from build123d import *

# Parameters (mm, degrees)
F1_DEPTH = 22
F3_DEPTH = 2
F5_DEPTH = 25
F7_DEPTH = 25


with BuildPart() as f1:
    # F0 (on Front) → F1 (new body, symmetric)
    with BuildSketch(Plane.XZ):
        with BuildLine():
            Line((-40, 0), (-0.4058661959, 0))
            ThreePointArc((-0.4058661959, 0), (-0.0297944203, 0.073409465), (0.2910628996, 0.2828599608))
            Line((0.2910628996, 0.2828599608), (1.7669371004, 1.7171400392))
            ThreePointArc((1.7669371004, 1.7171400392), (2.0877944203, 1.926590535), (2.4638661959, 2))
            Line((2.4638661959, 2), (26.037, 2))
            ThreePointArc((26.037, 2), (27.9687843496, 2.7891547709), (28.7954749436, 4.705176349))
            Line((28.7954749436, 4.705176349), (29.016465998, 16.0310205539))
            ThreePointArc((29.016465998, 16.0310205539), (28.8276722638, 16.8546583092), (28.2736767263, 17.4927109486))
            Line((28.2736767263, 17.4927109486), (27.3333525812, 18.1512658075))
            Line((27.3333525812, 18.1512658075), (26.1860444646, 16.5130704329))
            Line((26.1860444646, 16.5130704329), (26.8254471929, 16.0652655182))
            Line((26.8254471929, 16.0652655182), (26.037, 4))
            Line((26.037, 4), (1.4428661959, 4))
            ThreePointArc((1.4428661959, 4), (1.0667944203, 3.926590535), (0.7459371004, 3.7171400392))
            Line((0.7459371004, 3.7171400392), (-0.7299371004, 2.2828599608))
            ThreePointArc((-0.7299371004, 2.2828599608), (-1.0507944203, 2.073409465), (-1.4268661959, 2))
            Line((-1.4268661959, 2), (-40, 2))
            Line((-40, 2), (-40, 0))
        make_face()
    extrude(amount=F1_DEPTH, both=True)

    # F2 (on face) → F3 (join)
    with BuildSketch(Plane.XY.offset(2)):
        with BuildLine():
            Line((-50, 12), (-50, -12))
            ThreePointArc((-50, -12), (-47.0710678119, -19.0710678119), (-40, -22))
            Line((-40, -22), (-40, 22))
            ThreePointArc((-40, 22), (-47.0710678119, 19.0710678119), (-50, 12))
        make_face()
    extrude(amount=-F3_DEPTH)

    # F4 (on face) → F5 (cut)
    with BuildSketch(Plane.XY.offset(2)):
        with BuildLine():
            ThreePointArc((-40.35, -11.789), (-42.6, -14.039), (-40.35, -16.289))
            Line((-40.35, -16.289), (-20.35, -16.289))
            ThreePointArc((-20.35, -16.289), (-18.1, -14.039), (-20.35, -11.789))
            Line((-20.35, -11.789), (-40.35, -11.789))
        make_face()
        with BuildLine():
            ThreePointArc((-40.35, 16.289), (-42.6, 14.039), (-40.35, 11.789))
            Line((-40.35, 11.789), (-20.35, 11.789))
            ThreePointArc((-20.35, 11.789), (-18.1, 14.039), (-20.35, 16.289))
            Line((-20.35, 16.289), (-40.35, 16.289))
        make_face()
    extrude(amount=-F5_DEPTH, mode=Mode.SUBTRACT)

    # F6 (on face) → F7 (cut)
    with BuildSketch(Plane(origin=(28.6927430868, 0, -0.5598557981), x_dir=(0, 1, 0), z_dir=(0.9998096932, 0, -0.0195083911))):
        with BuildLine():
            Line((-9.9999997095, 13.096034309), (-17.9999997095, 13.096034309))
            ThreePointArc((-17.9999997095, 13.096034309), (-20, 11.0960344543), (-18, 9.096034309))
            Line((-18, 9.096034309), (-9.9999997095, 9.096034309))
            ThreePointArc((-9.9999997095, 9.096034309), (-7.9999997095, 11.096034309), (-9.9999997095, 13.096034309))
        make_face()
    extrude(amount=-F7_DEPTH, mode=Mode.SUBTRACT)


solid = f1.part
Check sheet for the modelled part. Datum: model origin and axes. Units: mm. A direction names the side the tool comes from. Give positions to 0.01 mm unless a question says otherwise; leave off trailing zeros. Loops run counter-clockwise (first coordinate to the right, second up) from the corner with the lowest first, then second, coordinate; pieces in that order, holes last. Notation, with made-up numbers: M -36,48.25 L -21,48.25 A24 ccw -21,67.25 Z; hole C -31.75,-11 d2. An arc over 180 degrees is marked long. Answer as a JSON object with one key per item and string values. Group by question number.
Q1. Cross-section at B-B on x = -41.5. Record the cut outline in (y, z).
Q2. Cross-section at A-A on y = 10. Record the cut outline in (x, z), then the cut area to 3 significant figures.
Q3. Access from +Z, -Z, +X, -X, +Y, -Y to the whole of each face (thin tool, end or side, straight path). Record for faces 5 (the flat face through (14, 0, 4)), 6 (the cylindrical face through (-42.6, -14, 1)).
Q4. Material ranges on line 1 along Y through (x, z) = (-25.5, 1.5); line 2 along Z through (x, y) = (19.5, 14); line 3 along Z through (x, y) = (-38, -18.5), recorded low to high. Write a range as [from, to].
Q5. Release check for a two-part mould opening along X. For faces 1 (the flat face through (-30, -11.789, 1)), 2 (the cylindrical face through (-46.99, 19.15, 1.01)), 3 (the flat face through (-26, 0, 2)), 4 (the cylindrical face through (28.833, -0.308, 16.844)) record: released by +X, released by -X, zero draft, split by the parting line, or undercut.
Q6. Cross-section at C-C on x = 20. Record the cut outline in (y, z).
Q7. Cross-section at D-D on z = 5.5. Record the cut outline in (x, y), then the cut area to 3 significant figures.
Q8. Go/stop test with flat-tipped pins: P1, Ø12, axis at x = 16.5, y = 6.5, coming from the -Z side; P2, Ø12, axis at x = -27, y = 6, coming from the +Z side; P3, Ø1.5, axis at x = 6.5, y = 11, coming from the +Z side. Record where each tip stops, or that it passes through.
Evaluation:
{
 "1": {"outline": "M -21.89,0 L -15.97,0 L -15.97,2 L -21.89,2 Z; M -12.11,0 L 12.11,0 L 12.11,2 L -12.11,2 Z; M 15.97,0 L 21.89,0 L 21.89,2 L 15.97,2 Z"},
 "2": {"outline": "M -50,0 L -0.41,0 A1 ccw 0.29,0.28 L 1.77,1.72 A1 cw 2.46,2 L 26.04,2 A2.76 ccw 28.8,4.71 L 29.02,16.03 A1.74 ccw 28.27,17.49 L 27.33,18.15 L 26.19,16.51 L 26.83,16.07 L 26.04,4 L 1.44,4 A1 ccw 0.75,3.72 L -0.73,2.28 A1 cw -1.43,2 L -50,2 Z", "area": "191 mm2"},
 "3": {"face 5": "+Z, -X, +Y, -Y", "face 6": "+Z, -Z"},
 "4": {"line 1": "y = [-22, -16.29], [-11.79, 11.79], [16.29, 22]", "line 2": "z = [2, 4]", "line 3": "z = [0, 2]"},
 "5": {"face 1": "undercut", "face 2": "released by -X", "face 3": "zero draft", "face 4": "released by +X"},
 "6": {"outline": "M -22,2 L 22,2 L 22,4 L -22,4 Z"},
 "7": {"outline": "M 26.14,-22 L 28.81,-22 L 28.81,22 L 26.14,22 Z", "area": "118 mm2"},
 "8": {"P1": "stops at z = 2", "P2": "stops at z = 2", "P3": "stops at z = 4"}
}
